For this review, take the finished solid that the model builds, in its own axes (mm). A direction names the side the tool comes from. Give positions to 0.01 mm unless a question says otherwise; leave off trailing zeros. Order: outer loops, then holes, each group sorted by start corner. A loop starts at its lowest first (then second) coordinate and runs counter-clockwise, first axis right, second up. Notation, with made-up numbers: (26, -3.75) - (61, -3.75) arc R28 ccw to (61, 26.25) - close; hole circle Ø3 at (4, 31). An arc over 180 degrees is marked (long way). One line per item, written item: value.
Autodesk Inventor part; units mm, degrees
ref_plane "YZ Plane" through (0, 0, 0) normal (1, 0, 0) x (0, 1, 0)
ref_plane "XZ Plane" through (0, 0, 0) normal (0, 1, 0) x (-1, 0, 0)
ref_plane "XY Plane" through (0, 0, 0) normal (0, 0, 1) x (1, 0, 0)
sketch "Sketch1" plane through (0, 0, 0) normal (0, 1, 0) x (-1, 0, 0)
  line L0 (0, 0) -> (22.5479, 0)
  line L1 (22.5089, -9.5249) -> (-0.0209, -9.5249)
  line L2 (-0.0209, -9.5249) -> (0, 0)
  arc A0 (22.5089, -9.5249) -> (22.5479, 0) centre (22.2912, -4.7615) ccw
  line L3 (0, 0) -> (-97.8508, -26.219)
  line L4 (0, 0) -> (101.3026, 0) construction
  line L5 (-97.8508, -26.219) -> (-95.3856, -35.4195)
  line L6 (0, 0) -> (2.4653, -9.2004)
  line L7 (2.4653, -9.2004) -> (-95.3856, -35.4195)
  circle A1 centre (22.2912, -4.7615) radius 2.2479
  line L8 (22.2912, -4.7615) -> (6.2892, -4.7615) construction
  circle A2 centre (6.2892, -4.7615) radius 2.2479
  line L9 (1.2326, -4.6002) -> (-11.0346, -7.8872) construction
  circle A3 centre (-11.0346, -7.8872) radius 1.9685
  line L10 (1.2326, -4.6002) -> (-96.6182, -30.8193) construction
  circle A4 centre (-20.4804, -10.4182) radius 1.9685
  circle A5 centre (-29.9262, -12.9492) radius 1.9685
  circle A6 centre (-39.372, -15.4802) radius 1.9685
  circle A7 centre (-48.8178, -18.0112) radius 1.9685
  circle A8 centre (-58.2636, -20.5422) radius 1.9685
  circle A9 centre (-67.7094, -23.0732) radius 1.9685
  circle A10 centre (-77.1552, -25.6042) radius 1.9685
  circle A11 centre (-86.6009, -28.1352) radius 1.9685
  line L11 (22.2912, -4.7615) -> (6.1685, -4.7615) construction
  line L12 (6.1685, -4.7615) -> (6.1685, 11.2405) construction
  line L13 (6.1685, 11.2405) -> (22.2912, 11.2405) construction
  line L14 (22.2912, 11.2405) -> (22.2912, -4.7615) construction
  line L15 (14.2299, 11.2405) -> (14.2299, -4.7615) construction
  line L16 (22.2912, 3.2395) -> (6.1685, 3.2395) construction
  circle A12 centre (14.2299, 3.2395) radius 1.27 construction
  dimension "d0" = 22.5298
  dimension "d1" = 9.525
  dimension "d2" = 4.7684
  dimension "d4" = 165
  dimension "d7" = 9.525
  dimension "d8" = 9.525
  dimension "d9" = 4.4958
  dimension "d10" = 16.002
  dimension "d11" = 4.4958
  dimension "d12" = 12.7
  dimension "d13" = 3.937
  dimension "d14" = 4.7625
  dimension "d15" = 3.937
  dimension "d16" = 9.779
  dimension "d17" = 3.937
  dimension "d18" = 9.779
  dimension "d19" = 3.937
  dimension "d20" = 9.779
  dimension "d21" = 3.937
  dimension "d22" = 9.779
  dimension "d23" = 3.937
  dimension "d24" = 9.779
  dimension "d25" = 3.937
  dimension "d26" = 9.779
  dimension "d27" = 3.937
  dimension "d28" = 9.779
  dimension "d29" = 3.937
  dimension "d30" = 9.779
  dimension "d31" = 16.002
  dimension "d32" = 2.54
  dimension "d33" = 115.8874
extrude "Extrusion1" add sketch "Sketch1" along normal blind 3.175
properties part number "CollectorArm165"
(1) Take a section at A-A (x = 67). Write out the cut boundary in (y, z) (3 decimals), then the cut area to 3 significant figures.
Answers below:
outline: (0, -27.814) - (3.175, -27.814) - (3.175, -24.909) - (0, -24.909) - close; (0, -21.237) - (3.175, -21.237) - (3.175, -17.953) - (0, -17.953) - close
area: 19.6 mm^2
(2) Machinability: for faces 1 (the face through (-4.5, 1.6, -3.4)), 2 (the face through (-12, 2, -9.525)), which of the approach directions +Z, -Z, +X, -X, +Y, -Y give a long, thin tool a straight path to every point of the face, cutting with its end or side? Answer none if there is none.
Answers below:
face 1: +Y, -Y
face 2: -Z, -X, +Y, -Y
(3) For P1, Ø4, axis at x = -22.29, z = -4.76, coming from the -Y side; P2, Ø1.6, axis at x = -8.5, y = 2, coming from the -Z side, all flat-tipped, find the tip position at first contact; note any pin that passes through.
Answers below:
P1: passes through
P2: stops at z = -9.52
(4) Draft analysis for pull direction Z (two halves, no side actions). For faces 3 (the face through (-27.06, 1.57, -4.68)), 4 (the face through (50.38, 1.565, -16.813)), 5 (the face through (36, 0, -16)), state which applies: pulls with the +Z half, pulls with the -Z half, needs draft (parallel to the pull), parting line crosses it, or undercut.
Answers below:
face 3: parting line crosses it
face 4: undercut
face 5: needs draft
(5) Take a section at C-C (x = -17.5). Write out the cut boundary in (y, z) (3 decimals), then the cut area to 3 significant figures.
Answers below:
outline: (0, -9.525) - (3.175, -9.525) - (3.175, 0) - (0, 0) - close
area: 30.2 mm^2
(6) Wall thickness on line 1 (Z direction, x = 22, y = 0.6); line 2 (Z direction, x = -19.5, y = 2.4); line 3 (Z direction, x = -5, y = 2.75): over which ranges is each line inside the solid? List them lowest first. Write a range as from..to.
Answers below:
line 1: z = -15.76..-11.67, -9.17..-5.89
line 2: z = -9.52..0
line 3: z = -9.52..-6.6, -2.92..0
(7) Take a section at D-D (x = 11). Write out the cut boundary in (y, z) (3 decimals), then the cut area to 3 significant figures.
Answers below:
outline: (0, -12.808) - (3.175, -12.808) - (3.175, -9.855) - (0, -9.855) - close; (0, -5.919) - (3.175, -5.919) - (3.175, -2.947) - (0, -2.947) - close
area: 18.8 mm^2
(8) Take a section at B-B (y = 1.8). Give the number of separate pieces and of enclosed holes in the cut face, then the cut area to 3 significant figures.
Answers below:
separate pieces: 1
enclosed holes: 11
area: 1,060 mm^2
